```python
from build123d import *

# Parameters (mm, degrees)
SKETCH1_R           = 2.159
BOSS_EXTRUDE1_DEPTH = 3.175


with BuildPart() as part:
    # Sketch1 → Boss-Extrude1 (new, symmetric)
    with BuildSketch(Plane.XY):
        with BuildLine():
            Line((56.212406906, 19.490008209), (12.807859934, 21.061903429))
            ThreePointArc((12.807859934, 21.061903429), (1.486348152, 17.419283948), (-4.876850173, 7.371646773))
            Line((-4.876850173, 7.371646773), (-6.200989145, 1.36756485))
            ThreePointArc((-6.200989145, 1.36756485), (-1.36756485, -6.200989145), (6.200989145, -1.36756485))
            Line((6.200989145, -1.36756485), (7.525128118, 4.636517072))
            ThreePointArc((7.525128118, 4.636517072), (9.126161655, 7.268805354), (12.003509079, 8.370223433))
            Line((12.003509079, 8.370223433), (56.212406906, 9.971248211))
            ThreePointArc((56.212406906, 9.971248211), (60.802546008, 14.73062821), (56.212406906, 19.490008209))
        make_face()
        Circle(SKETCH1_R, mode=Mode.SUBTRACT)
        with Locations((56.040046008, 14.73062821)):
            Circle(SKETCH1_R, mode=Mode.SUBTRACT)
    extrude(amount=BOSS_EXTRUDE1_DEPTH, both=True)


solid = part.part
```
Work out the finished part from the listing and answer in its coordinate system (mm). Give positions to 0.01 mm unless a question says otherwise; leave off trailing zeros. Write each loop counter-clockwise with the first axis right and the second up, starting at its lowest first coordinate (ties: lowest second). Pieces come first, ordered by that corner, then holes. Notation, with made-up numbers: (44, 65) -> (95, 65) arc R19 ccw to (95, 100) -> close; hole circle Ø3 at (0, 75). An arc over 180 degrees is marked (long way). Write each question's results on one line, items separated by ' | '.
1. Find section D-D on y = 5.25. Determine the outline of the cut face in (x, z) (3 decimals), and give its area (3 significant figures).
Data:
outline: (-5.345, -3.175) -> (7.704, -3.175) -> (7.704, 3.175) -> (-5.345, 3.175) -> close | area: 82.9 mm^2
2. Each of these flat-tipped pins is pushed along its axis until it touches: pin 1 Ø2 at (y, z) = (7, -1.5) entering from -X; pin 2 Ø10 at (x, y) = (45, 3.5) entering from -Z. Where does it stop, or does it pass through?
Data:
pin 1: x = -5.18 | pin 2: through
3. Determine the mould class of faces 1 (the cylindrical face through (60.8, 14.6, 0)), 2 (the cylindrical face through (1.62, 17.52, 0.04)), 3 (the cylindrical face through (58.034, 13.904, -0.044)), 4 (the cylindrical face through (-0.28, 2.14, -0.04)) for opening direction Y: +Y half, -Y half, draft (parallel to the pull), parting line (faces both ways), or undercut.
Data:
face 1: parting line | face 2: +Y half | face 3: undercut | face 4: undercut
4. Find section C-C on z = 1.5. Give the number of separate pieces and of enclosed holes in the cut face, and give its area (3 significant figures).
Data:
separate pieces: 1 | enclosed holes: 2 | area: 827 mm^2
5. Find section A-A on x = 0. Determine the outline of the cut face in (y, z) (3 decimals).
Data:
outline: (-6.35, -3.175) -> (-2.159, -3.175) -> (-2.159, 3.175) -> (-6.35, 3.175) -> close; (2.159, -3.175) -> (16.128, -3.175) -> (16.128, 3.175) -> (2.159, 3.175) -> close
6. Straight lines are drawn through the part: L1, parallel to Y at x = 0, z = 0; L2, parallel to X at y = 1, z = -2.5; L3, parallel to X at y = 16.5, z = -1.75. For each, find the intervals that lie inside material, in ascending order.
Data:
L1: -6.35 to -2.16, 2.16 to 16.13 | L2: -6.27 to -1.91, 1.91 to 6.72 | L3: 0.39 to 54.8, 57.28 to 60.46
7. Find section B-B on y = 15.5. Determine the outline of the cut face in (x, z) (3 decimals), and give its area (3 significant figures).
Data:
outline: (-0.614, -3.175) -> (54.023, -3.175) -> (54.023, 3.175) -> (-0.614, 3.175) -> close; (58.057, -3.175) -> (60.74, -3.175) -> (60.74, 3.175) -> (58.057, 3.175) -> close | area: 364 mm^2
